Check sheet for the drawn part. Datum: minimum x, y, z corner. Units: mm. A direction names the side the tool comes from. Coordinates: 2 decimals unless noted, no trailing zeros. Loops run counter-clockwise (first coordinate to the right, second up) from the corner with the lowest first, then second, coordinate; pieces in that order, holes last.
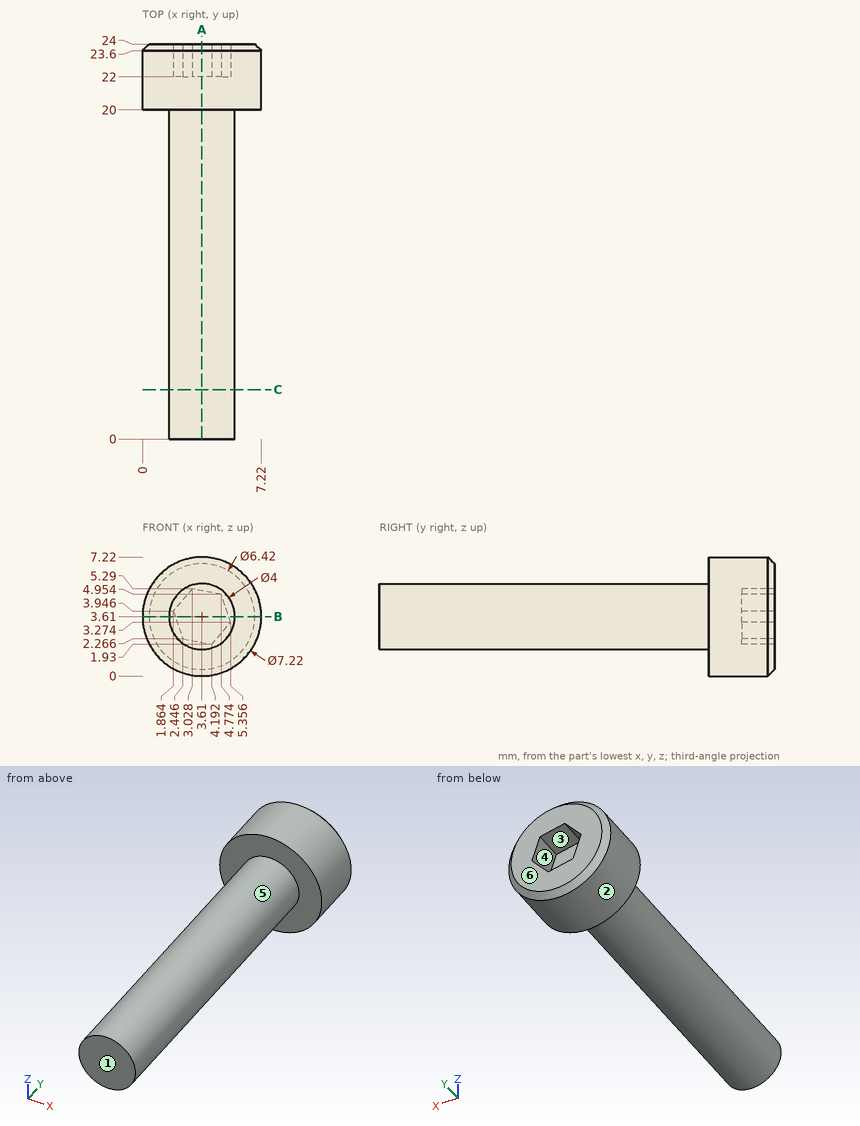
(1) Sectioned sample at C-C on y = 3. Record the cut outline in (x, z).
Findings:
outline: circle Ø4 at (3.61, 3.61)
(2) Access from +Z, -Z, +X, -X, +Y, -Y to the whole of each face (thin tool, end or side, straight path). Record for the marked faces 4, 5 and 6.
Findings:
face 4: +Y
face 5: -Y
face 6: +Z, -Z, +X, -X, +Y
(3) Gauge pin test, flat ends, axial feed: pin 1 Ø2 at (y, z) = (10, 3) entering from +X; pin 2 Ø1 at (x, z) = (3.5, 4) entering from +Y; pin 3 Ø1 at (x, y) = (2, 3) entering from +Z. Record the tip position at first contact, or that the pin passes through.
Findings:
pin 1: stops at x = 5.61
pin 2: stops at y = 22
pin 3: stops at z = 5.27
(4) Draft check along X on the marked faces 1, 2 and 3. Enter one of: +X half, -X half, draft (parallel to the pull), parting line (faces both ways), or undercut.
Findings:
face 1: draft
face 2: parting line
face 3: undercut
(5) Sectioned sample at A-A on x = 3.61. Record the cut outline in (y, z).
Findings:
outline: (0, 1.61) - (20, 1.61) - (20, 0) - (23.6, 0) - (24, 0.4) - (24, 2.04) - (22, 2.04) - (22, 5.18) - (24, 5.18) - (24, 6.82) - (23.6, 7.22) - (20, 7.22) - (20, 5.61) - (0, 5.61) - close
(6) Scan lines: L1, parallel to Y at x = 2.25, z = 1.5; L2, parallel to Y at x = 3, z = 2.75; L3, parallel to X at y = 19, z = 3.5. Record each from-to range of solid material in increasing order.
Findings:
L1: y = 20 to 24
L2: y = 0 to 22
L3: x = 1.61 to 5.61
(7) Sectioned sample at B-B on z = 3.61. Record the cut outline in (x, y), and give its area (3 significant figures).
Findings:
outline: (0, 20) - (1.61, 20) - (1.61, 0) - (5.61, 0) - (5.61, 20) - (7.22, 20) - (7.22, 23.6) - (6.82, 24) - (5.24, 24) - (5.24, 22) - (1.98, 22) - (1.98, 24) - (0.4, 24) - (0, 23.6) - close
area: 102 mm2
